The listing builds one solid part. Answer for the finished solid, in the listing's coordinates (mm). A direction names the side the tool comes from. Round coordinates to 2 decimals unless told otherwise and drop trailing zeros. Order: outer loops, then holes, each group sorted by start corner. A loop starts at its lowest first (then second) coordinate and runs counter-clockwise, first axis right, second up. Notation, with made-up numbers: (4, 51) - (19, 51) arc R16 cw to (19, 74) - close; hole circle Ø9 at (43.25, 57). An arc over 180 degrees is marked (long way). One line per item, written item: value. Start each with the question number.
1. Section B-B, the plane y = 9 is taken. Give the vertices of the cut face in (x, z).
2. A tool of negligible diameter and unlimited length cuts with its end or side. For faces 1 (the flat face through (0, 15, -8)), 2 (the flat face through (-17, 14.3, 0)), 3 (the cylindrical face through (-21.495, 7.933, -0.473)), 4 (the flat face through (13.8, 15, 0)), 5 (the cylindrical face through (-1.464, 3.451, 0.325)), from which of +Z, -Z, +X, -X, +Y, -Y can it reach the whole face along a straight path? Write none if from no direction.
3. For a pull along Z with two mould halves and no side action, classify faces 6 (the flat face through (0.3, 2, -23.5)), 7 (the flat face through (17, 14.3, 0)), 8 (the cylindrical face through (12.957, 8.366, -0.651)) as released by +Z, released by -Z, zero draft, split by the parting line, or undercut.
4. Section C-C, the plane x = -8 is taken. Give the vertices of the cut face in (y, z).
5. Section A-A, the plane z = 0 is taken. Count the separate pieces of the cut face and the enclosed holes in it, then the cut area to 3 significant figures.
6. Straight lines are drawn through the part: line 1 (X direction, y = 9.25, z = 0); line 2 (X direction, y = 5.5, z = 0); line 3 (Y direction, x = -20, z = 13). For each, find the intervals that lie inside material, in ascending order.
7. Flat-ended cylindrical pins translate along their axes: P1, Ø5, axis at x = -19, y = 13, coming from the -Z side; P2, Ø0.8, axis at x = 0, y = 13.5, coming from the -Z side; P3, Ø3, axis at y = 2, z = -18.5, coming from the -X side. Find the tip coordinate at first contact, or state that the pin passes through.
8. Section D-D, the plane z = 17.5 is taken. Give the vertices of the cut face in (x, y).
from build123d import *
from build123d.topology import SkipClean

# Parameters (mm, degrees)
SKETCH1_R                            = 30
BOSS_EXTRUDE1_DEPTH                  = 4
BOSS_EXTRUDE2_REACH                  = 44.615
BOSS_EXTRUDE2_END_RADIUS             = 30
BOSS_EXTRUDE2_DIRECTION_2_REACH      = 44.615
BOSS_EXTRUDE2_DIRECTION_2_END_RADIUS = 30
SKETCH3_OUTSIDE_W                    = 78.092
SKETCH3_OUTSIDE_H                    = 69.092
SKETCH3_OUTSIDE_R                    = 21.5
CUT_EXTRUDE2_DEPTH                   = 12.5
BOSS_EXTRUDE3_DEPTH                  = 18
BOSS_EXTRUDE4_DEPTH                  = 15
BOSS_EXTRUDE5_DEPTH                  = 15
CUT_EXTRUDE3_DEPTH                   = 44.292609069
CUT_EXTRUDE3_DEPTH_BACK              = 44.292609069
SKETCH8_R                            = 2
CUT_EXTRUDE8_DEPTH                   = 48.077064479
CUT_EXTRUDE8_DEPTH_BACK              = 48.077064479
CUT_EXTRUDE9_DEPTH                   = 59.659818207
CUT_EXTRUDE11_DEPTH                  = 20
CUT_EXTRUDE12_DEPTH                  = 20
CUT_EXTRUDE13_DEPTH                  = 20
CUT_EXTRUDE14_DEPTH                  = 44.292609069
CUT_EXTRUDE14_DEPTH_BACK             = 44.292609069
SKETCH25_W                           = 66.075437062
SKETCH25_H                           = 20.142243048
SKETCH26_R                           = 5
CUT_EXTRUDE15_DEPTH                  = 24
CUT_EXTRUDE17_DEPTH                  = 47.524187258
CUT_EXTRUDE17_DEPTH_BACK             = 47.524187258
SKETCH29_W                           = 7.7
SKETCH29_H                           = 2.2
CUT_EXTRUDE18_DEPTH                  = 47.524187258
CUT_EXTRUDE18_DEPTH_BACK             = 47.524187258
SKETCH31_W                           = 7.7
SKETCH31_H                           = 2.2
CUT_EXTRUDE20_DEPTH                  = 43.690748412
CUT_EXTRUDE20_DEPTH_BACK             = 43.690748412
SKETCH33_R                           = 2.5
SKETCH34_R                           = 1.5
CUT_EXTRUDE21_DEPTH                  = 10
SKETCH35_W                           = 2.6
SKETCH35_H                           = 16
CUT_EXTRUDE23_DEPTH                  = 4
BOSS_EXTRUDE6_REACH                  = 45.614
SKETCH37_R                           = 1


with BuildPart() as part:
    # Sketch1 → Boss-Extrude1 (new body)
    with BuildSketch(Plane(origin=(0, 0, 0), x_dir=(1, 0, 0), z_dir=(0, 1, 0))):
        with Locations(Location((0, 0, 0), (0, 0, 270))):
            Circle(SKETCH1_R)
    extrude(amount=BOSS_EXTRUDE1_DEPTH)

    # Boss-Extrude2: up to this cylinder (the profile starts inside it)
    with SkipClean():  # the faces are left unmerged after this step: merging them gives an invalid solid
        boss_extrude2_end = Plane(origin=(0, 9.396175, 0), z_dir=(0, -1, 0)) * Cylinder(BOSS_EXTRUDE2_END_RADIUS, 150.23, mode=Mode.PRIVATE)
        # Sketch2 → Boss-Extrude2 (add, up to the surface)
        with BuildSketch(Plane(origin=(0, 0, 0), x_dir=(0, 0, -1), z_dir=(1, 0, 0)), mode=Mode.PRIVATE) as boss_extrude2_sk1:
            Polygon((0, 4), (21.5, 4), (9, 16.5), (-9, 16.5), (-21.5, 4), align=None)
        boss_extrude2_tool1 = extrude(boss_extrude2_sk1.sketch, amount=BOSS_EXTRUDE2_REACH, mode=Mode.PRIVATE) & boss_extrude2_end
        add(boss_extrude2_tool1.solids().sort_by_distance((0, 9.396175, 0))[0])

    # Boss-Extrude2 direction 2: up to this cylinder (the profile starts inside it)
    with SkipClean():  # the faces are left unmerged after this step: merging them gives an invalid solid
        boss_extrude2_direction_2_end = Plane(origin=(0, 9.396175, 0), z_dir=(0, -1, 0)) * Cylinder(BOSS_EXTRUDE2_DIRECTION_2_END_RADIUS, 150.23, mode=Mode.PRIVATE)
        # Sketch2 → Boss-Extrude2 direction 2 (add, up to the surface)
        with BuildSketch(Plane(origin=(0, 0, 0), x_dir=(0, 0, -1), z_dir=(1, 0, 0)), mode=Mode.PRIVATE) as boss_extrude2_direction_2_sk1:
            Polygon((0, 4), (21.5, 4), (9, 16.5), (-9, 16.5), (-21.5, 4), align=None)
        boss_extrude2_direction_2_tool1 = extrude(boss_extrude2_direction_2_sk1.sketch, amount=-BOSS_EXTRUDE2_DIRECTION_2_REACH, mode=Mode.PRIVATE) & boss_extrude2_direction_2_end
        add(boss_extrude2_direction_2_tool1.solids().sort_by_distance((0, 9.396175, 0))[0])

    # SurfaceCut1
    split(bisect_by=Plane(origin=(0, 12.75, -12.75), x_dir=(1, 0, 0), z_dir=(0, 0.7071067811865558, -0.7071067811865392)), keep=Keep.BOTTOM)

    # SurfaceCut2
    split(bisect_by=Plane(origin=(0, 12.75, 12.75), x_dir=(1, 0, 0), z_dir=(0, 0.7071067811865509, 0.7071067811865442)), keep=Keep.BOTTOM)

    # Sketch3 outside → Cut-Extrude2 (cut)
    with BuildSketch(Plane(origin=(0, 4, 0), x_dir=(1, 0, 0), z_dir=(0, 1, 0))):
        Rectangle(SKETCH3_OUTSIDE_W, SKETCH3_OUTSIDE_H)
        Circle(SKETCH3_OUTSIDE_R, mode=Mode.SUBTRACT)
    extrude(amount=CUT_EXTRUDE2_DEPTH, mode=Mode.SUBTRACT)

    # Sketch5 → Boss-Extrude3 (add)
    with BuildSketch(Plane(origin=(0, 0, 0), x_dir=(-1, 0, 0), z_dir=(0, -1, 0))):
        Polygon((0, -6), (-17.5, -6), (-17.5, 6), (17.5, 6), (17.5, -6), align=None)
    extrude(amount=BOSS_EXTRUDE3_DEPTH)

    # Sketch6 → Boss-Extrude4 (add)
    with BuildSketch(Plane.XZ):
        Polygon((0, 15), (7, 15), (7, 6), (-7, 6), (-7, 15), align=None)
    extrude(amount=BOSS_EXTRUDE4_DEPTH)

    # Sketch7 → Boss-Extrude5 (add)
    with BuildSketch(Plane.XZ):
        Polygon((0, -15), (7, -15), (7, -6), (-7, -6), (-7, -15), align=None)
    extrude(amount=BOSS_EXTRUDE5_DEPTH)

    # Sketch8 → Cut-Extrude3 (cut, two sides: drawn at the far end of the back side and taken through both)
    with BuildSketch(Plane.XY.offset(-CUT_EXTRUDE3_DEPTH_BACK)):
        with Locations((-12.5, -12.5)):
            Circle(SKETCH8_R)
        with Locations((12.5, -12.5)):
            Circle(SKETCH8_R)
    extrude(amount=CUT_EXTRUDE3_DEPTH + CUT_EXTRUDE3_DEPTH_BACK, mode=Mode.SUBTRACT)

    # Sketch16 → Cut-Extrude8 (cut, two sides: drawn at the far end of the back side and taken through both)
    with BuildSketch(Plane.XY.offset(6).offset(-CUT_EXTRUDE8_DEPTH_BACK)):
        Polygon((17.5, -18), (17.5, -14.5), (14, -18), align=None)
        Polygon((-17.5, -18), (-14, -18), (-17.5, -14.5), align=None)
    extrude(amount=CUT_EXTRUDE8_DEPTH + CUT_EXTRUDE8_DEPTH_BACK, mode=Mode.SUBTRACT)

    # Sketch17 → Cut-Extrude9 (cut, through all)
    with BuildSketch(Plane(origin=(10.365975269, -9.674910251, -8.062425209), x_dir=(-0.3613483622370374, 0.337258471421235, -0.8693009171531012), z_dir=(0.6355070151731325, -0.5931398808282571, -0.49428323402354774))):
        Polygon((-2.372510104, -6.189601271), (7.980636686, -0.706686759), (7.980636686, -10.965829024), align=None)
    extrude(amount=CUT_EXTRUDE9_DEPTH, mode=Mode.SUBTRACT)

    # Sketch19 → Cut-Extrude11 (cut)
    with BuildSketch(Plane(origin=(-10.365975269, -9.674910251, -8.062425209), x_dir=(0.3613483622370374, 0.33725847142123494, -0.8693009171531012), z_dir=(0.6355070151731324, 0.5931398808282571, 0.4942832340235476))):
        Polygon((-2.372510104, -6.189601271), (7.980636686, -10.965829024), (7.980636686, -0.706686759), align=None)
    extrude(amount=-CUT_EXTRUDE11_DEPTH, mode=Mode.SUBTRACT)

    # Sketch20 → Cut-Extrude12 (cut)
    with BuildSketch(Plane(origin=(-10.365975269, -9.674910251, 8.062425209), x_dir=(-0.3613483622370374, -0.3372584714212349, -0.8693009171531013), z_dir=(0.6355070151731326, 0.593139880828257, -0.49428323402354757))):
        Polygon((2.372510104, -6.189601271), (-7.980636686, -0.706686759), (-7.980636686, -10.965829024), align=None)
    extrude(amount=-CUT_EXTRUDE12_DEPTH, mode=Mode.SUBTRACT)

    # Sketch21 → Cut-Extrude13 (cut)
    with BuildSketch(Plane(origin=(10.365975269, -9.674910251, 8.062425209), x_dir=(-0.3613483622370374, 0.3372584714212349, 0.8693009171531013), z_dir=(-0.6355070151731326, 0.593139880828257, -0.49428323402354757))):
        Polygon((-2.372510104, -6.189601271), (7.980636686, -0.706686759), (7.980636686, -10.965829024), align=None)
    extrude(amount=-CUT_EXTRUDE13_DEPTH, mode=Mode.SUBTRACT)

    # Sketch25 → Cut-Extrude14 (cut, two sides: drawn at the far end of the back side and taken through both)
    with BuildSketch(Plane.XY.offset(-CUT_EXTRUDE14_DEPTH_BACK)):
        with Locations((0, -10.071121524)):
            Rectangle(SKETCH25_W, SKETCH25_H)
    extrude(amount=CUT_EXTRUDE14_DEPTH + CUT_EXTRUDE14_DEPTH_BACK, mode=Mode.SUBTRACT)

    # Sketch26 → Cut-Extrude15 (cut)
    with BuildSketch(Plane(origin=(0, 16.5, 0), x_dir=(1, 0, 0), z_dir=(0, 1, 0))):
        with Locations(Location((-8, 0, 0), (0, 0, 270))):
            Circle(SKETCH26_R)
        with Locations(Location((8, 0, 0), (0, 0, 270))):
            Circle(SKETCH26_R)
    extrude(amount=-CUT_EXTRUDE15_DEPTH, mode=Mode.SUBTRACT)

    # Sketch29 → Cut-Extrude17 (cut, two sides: drawn at the far end of the back side and taken through both)
    with BuildSketch(Plane.XY.offset(6).offset(-CUT_EXTRUDE17_DEPTH_BACK)):
        with Locations((17.65, 15.4)):
            Rectangle(SKETCH29_W, SKETCH29_H)
    extrude(amount=CUT_EXTRUDE17_DEPTH + CUT_EXTRUDE17_DEPTH_BACK, mode=Mode.SUBTRACT)

    # Sketch31 → Cut-Extrude18 (cut, two sides: drawn at the far end of the back side and taken through both)
    with BuildSketch(Plane.XY.offset(6).offset(-CUT_EXTRUDE18_DEPTH_BACK)):
        with Locations((-17.65, 15.4)):
            Rectangle(SKETCH31_W, SKETCH31_H)
    extrude(amount=CUT_EXTRUDE18_DEPTH + CUT_EXTRUDE18_DEPTH_BACK, mode=Mode.SUBTRACT)

    # Sketch33 → Cut-Extrude20 (cut, two sides: drawn at the far end of the back side and taken through both)
    with BuildSketch(Plane.XY.offset(-CUT_EXTRUDE20_DEPTH_BACK)):
        with Locations(Location((0, 9, 0), (0, 0, 270))):
            Circle(SKETCH33_R)
    extrude(amount=CUT_EXTRUDE20_DEPTH + CUT_EXTRUDE20_DEPTH_BACK, mode=Mode.SUBTRACT)

    # Sketch34 → Cut-Extrude21 (cut)
    with BuildSketch(Plane.XZ):
        with Locations(Location((0, 0, 0), (0, 0, 270))):
            Circle(SKETCH34_R)
    extrude(amount=-CUT_EXTRUDE21_DEPTH, mode=Mode.SUBTRACT)

    # Sketch35 → Cut-Extrude23 (cut)
    with BuildSketch(Plane(origin=(0, 16.5, 0), x_dir=(1, 0, 0), z_dir=(0, 1, 0))):
        Rectangle(SKETCH35_W, SKETCH35_H)
    extrude(amount=-CUT_EXTRUDE23_DEPTH, mode=Mode.SUBTRACT)

    # Sketch37 → Boss-Extrude6 (add, up to next)
    with BuildSketch(Plane(origin=(-1.3, 0, 0), x_dir=(0, 0, -1), z_dir=(1, 0, 0)), mode=Mode.PRIVATE) as boss_extrude6_sk1:
        with Locations(Location((-5, 14.5, 0), (0, 0, 180))):
            Circle(SKETCH37_R)
    boss_extrude6_tool1 = extrude(boss_extrude6_sk1.sketch, amount=BOSS_EXTRUDE6_REACH, mode=Mode.PRIVATE) - part.part
    # Sketch37 → Boss-Extrude6 (add, up to next)
    with BuildSketch(Plane(origin=(-1.3, 0, 0), x_dir=(0, 0, -1), z_dir=(1, 0, 0)), mode=Mode.PRIVATE) as boss_extrude6_sk2:
        with Locations(Location((0, 14.5, 0), (0, 0, 180))):
            Circle(SKETCH37_R)
    boss_extrude6_tool2 = extrude(boss_extrude6_sk2.sketch, amount=BOSS_EXTRUDE6_REACH, mode=Mode.PRIVATE) - part.part
    # Sketch37 → Boss-Extrude6 (add, up to next)
    with BuildSketch(Plane(origin=(-1.3, 0, 0), x_dir=(0, 0, -1), z_dir=(1, 0, 0)), mode=Mode.PRIVATE) as boss_extrude6_sk3:
        with Locations(Location((5, 14.5, 0), (0, 0, 180))):
            Circle(SKETCH37_R)
    boss_extrude6_tool3 = extrude(boss_extrude6_sk3.sketch, amount=BOSS_EXTRUDE6_REACH, mode=Mode.PRIVATE) - part.part
    add(boss_extrude6_tool1.solids().sort_by_distance((-1.3, 14.5, 5))[0])
    add(boss_extrude6_tool2.solids().sort_by_distance((-1.3, 14.5, 0))[0])
    add(boss_extrude6_tool3.solids().sort_by_distance((-1.3, 14.5, -5))[0])


solid = part.part
Answer list:
1. outline: (-13.78, -16.5) - (-2.5, -16.5) - (-2.5, 16.5) - (-13.78, 16.5) arc R21.5 ccw to start; (2.5, -16.5) - (13.78, -16.5) arc R21.5 ccw to (13.78, 16.5) - (2.5, 16.5) - close; hole circle Ø10 at (-8, 0); hole circle Ø10 at (8, 0)
2. face 1: +Y
2. face 2: +Z, -Z, -X, +Y
2. face 3: -X, +Y
2. face 4: +Z, -Z, +X, +Y
2. face 5: -Y
3. face 6: released by -Z
3. face 7: zero draft
3. face 8: undercut
4. outline: (0, -25.5) - (4, -21.5) - (4, -19.96) - (5.54, -19.96) - (16.5, -9) - (16.5, -5) - (0, -5) - close; (0, 5) - (16.5, 5) - (16.5, 9) - (5.54, 19.96) - (4, 19.96) - (4, 21.5) - (0, 25.5) - close
5. separate pieces: 3
5. enclosed holes: 1
5. area: 369 mm²
6. line 1: x = -21.5 to -13, -3 to -2.49, 2.49 to 3, 13 to 21.5
6. line 2: x = -21.5 to -13, -3 to -1.5, 1.5 to 3, 13 to 21.5
6. line 3: y = 0 to 4
7. P1: stops at z = -13.52
7. P2: stops at z = -12.4
7. P3: stops at x = -24.72
8. outline: (-24.37, 0) - (24.37, 0) - (24.37, 4) - (12.49, 4) - (12.49, 8) - (2.29, 8) arc R2.5 cw to (-2.29, 8) - (-12.49, 8) - (-12.49, 4) - (-24.37, 4) - close
